Source: CAD feature listing. Evaluate the final solid. Frame: model axes, mm. Round coordinates to 2 decimals unless told otherwise and drop trailing zeros. Loops run counter-clockwise (first coordinate to the right, second up) from the corner with the lowest first, then second, coordinate; pieces in that order, holes last.
Item 1: Section query A-A on z = 0.5. Return loops of the section in (x, y).
Item 2: Pull-direction query (Z, two-part tool) for faces 1 (the flat face through (99, 13, 1.59)), 2 (the flat face through (99, 13, -1.59)); classes: released by +Z, released by -Z, zero draft, split by the parting line, or undercut.
Item 3: First-contact query: P1, Ø1.6, axis at y = 21, z = 0, coming from the +X side; P2, Ø1.6, axis at y = 1.5, z = 0.5, coming from the -X side. Flat tips, straight axial feed; report the tip coordinate or a pass-through.
Item 4: Section query B-B on y = 1.75. Return loops of the section in (x, z), then the cut area to 3 significant figures.
Item 5: Ray query, L1, parallel to Y at x = 117.5, z = 1; L2, parallel to X at y = 16.25, z = 0.05; L3, parallel to Y at x = 108, z = 0.75. Return the intervals inside material, ascending.
```python
from build123d import *

# Parameters (mm, degrees)
SKETCH2_W           = 200
SKETCH2_H           = 25
BOSS_EXTRUDE1_DEPTH = 1.59
SKETCH4_R           = 1
SKETCH4_W           = 23
SKETCH4_H           = 12.1
CUT_EXTRUDE1_DEPTH  = 3.18
SKETCH5_W           = 6.36
SKETCH5_H           = 12.5
BOSS_EXTRUDE2_DEPTH = 3.18


with BuildPart() as part:
    # Sketch2 → Boss-Extrude1 (new, symmetric)
    with BuildSketch(Plane.XY):
        with Locations((100, 12.5)):
            Rectangle(SKETCH2_W, SKETCH2_H)
    extrude(amount=BOSS_EXTRUDE1_DEPTH, both=True)

    # Sketch4 → Cut-Extrude1 (cut)
    with BuildSketch(Plane(origin=(0, 0, -1.59), x_dir=(-1, 0, 0), z_dir=(0, 0, -1))):
        with Locations((-135, 12.457546073)):
            Circle(SKETCH4_R)
        with Locations((-108, 12.457546073)):
            Circle(SKETCH4_R)
        with Locations((-121.5, 12.457546073)):
            Rectangle(SKETCH4_W, SKETCH4_H)
    extrude(amount=-CUT_EXTRUDE1_DEPTH, mode=Mode.SUBTRACT)

    # Sketch5 → Boss-Extrude2 (add)
    with BuildSketch(Plane(origin=(0, 0, -1.59), x_dir=(-1, 0, 0), z_dir=(0, 0, -1))):
        with Locations((-203.18, 12.5)):
            Rectangle(SKETCH5_W, SKETCH5_H)
        with Locations((3.18, 12.5)):
            Rectangle(SKETCH5_W, SKETCH5_H)
    extrude(amount=-BOSS_EXTRUDE2_DEPTH)


solid = part.part
```
Data:
1. outline: (-6.36, 6.25) - (0, 6.25) - (0, 0) - (200, 0) - (200, 6.25) - (206.36, 6.25) - (206.36, 18.75) - (200, 18.75) - (200, 25) - (0, 25) - (0, 18.75) - (-6.36, 18.75) - close; hole circle Ø2 at (108, 12.46); hole (110, 6.41) - (133, 6.41) - (133, 18.51) - (110, 18.51) - close; hole circle Ø2 at (135, 12.46)
2. face 1: released by +Z
2. face 2: released by -Z
3. P1: stops at x = 200
3. P2: stops at x = 0
4. outline: (0, -1.59) - (200, -1.59) - (200, 1.59) - (0, 1.59) - close
4. area: 636 mm2
5. L1: y = 0 to 6.41, 18.51 to 25
5. L2: x = -6.36 to 110, 133 to 206.36
5. L3: y = 0 to 11.46, 13.46 to 25
